from build123d import *

# Parameters (mm, degrees)
F0_W     = 70
F0_H     = 152.653071
F0_W_2   = 50.857146
F0_H_2   = 65.091088
F1_DEPTH = 8
F2_D     = 2
F2_DEPTH = 50
F3_R     = 10


with BuildPart() as f1:
    # F0 (on Top) → F1 (new body)
    with BuildSketch(Plane.XY):
        with Locations((0, 0.142402)):
            Rectangle(F0_W, F0_H)
        with Locations((0, -36.596865)):
            Rectangle(F0_W_2, F0_H_2, mode=Mode.SUBTRACT)
        with Locations((0, 36.596865)):
            Rectangle(F0_W_2, F0_H_2, mode=Mode.SUBTRACT)
    extrude(amount=F1_DEPTH)

    # F2
    with Locations(Plane(origin=(0, 0, 0), x_dir=(1, 0, 0), z_dir=(0, 0, -1))):
        with Locations((0, 2), (0, -2), (0, 73.713833), (0, -73.713833)):
            Hole(F2_D / 2, depth=F2_DEPTH)

    # F3
    f3_edges = [f1.edges().sort_by_distance(p)[0] for p in [
        (-35, 76.468938, 4),
        (35, 76.468938, 4),
        (-35, -76.184133, 4),
        (35, -76.184133, 4),
    ]]
    fillet(f3_edges, radius=F3_R)


solid = f1.part
Build history of the part. All positions in model axes, mm. A direction names the side the tool comes from. Round coordinates to 2 decimals unless told otherwise and drop trailing zeros. Write each loop counter-clockwise with the first axis right and the second up, starting at its lowest first coordinate (ties: lowest second). Pieces come first, ordered by that corner, then holes. Notation, with made-up numbers: M 58.5,-10.5 L 71.5,-10.5 A17 ccw 71.5,3.5 Z; hole C 34.25,-12.5 d5. An arc over 180 degrees is marked long. Answer as a JSON object with one key per item and string values. Group by question number.
(1) Which spindle directions (+Z, -Z, +X, -X, +Y, -Y) get a long thin tool onto all of the face, cutting with end or side? Do faces 4 (the flat face through (-25.429, -37, 4)), 5 (the flat face through (-35, -1, 4)). Say none if no direction does.
(2) Cut at A-A (y = 63). Give the cut face in (x, z).
(3) Flat gauge pin, fed straight in: pin 1 (12 mm diameter, centred on x = -15.5, y = 28.5, fed in from -Z). Where does the tip first touch, or does it go through?
(4) Cut at C-C (z = 2). Give the cut face in (x, y), and give its area (3 significant figures).
(5) Cut at D-D (x = 31.5). Give the cut face in (y, z), and give its area (3 significant figures).
(6) Drill centre lines: L1, parallel to Y at x = -7.5, z = 0.5; L2, parallel to X at y = 62, z = 7.5; L3, parallel to Y at x = 31, z = 4.25. Where is each one in solid material? Low to high.
(7) Mould opens along Y. For faces 1 (the flat face through (0, 4.051, 4)), 2 (the cylindrical face through (-32.15, 73.46, 4.06)), 3 (the flat face through (-3, 0, 0)) say: pulls with the +Y half, pulls with the -Y half, needs draft (parallel to the pull), parting line crosses it, or undercut.
(8) Cut at B-B (x = 14). Give the cut face in (y, z).
Responses:
{
 "1": {"face 4": "+Z, -Z", "face 5": "+Z, -Z, -X, +Y, -Y"},
 "2": {"outline": "M -35,0 L -25.43,0 L -25.43,8 L -35,8 Z; M 25.43,0 L 35,0 L 35,8 L 25.43,8 Z"},
 "3": {"pin 1": "passes through"},
 "4": {"outline": "M -35,-66.18 A10 ccw -25,-76.18 L 25,-76.18 A10 ccw 35,-66.18 L 35,66.47 A10 ccw 25,76.47 L -25,76.47 A10 ccw -35,66.47 Z; hole M -25.43,-69.14 L 25.43,-69.14 L 25.43,-4.05 L -25.43,-4.05 Z; hole M -25.43,4.05 L 25.43,4.05 L 25.43,69.14 L -25.43,69.14 Z; hole C 0,-73.71 d2; hole C 0,-2 d2; hole C 0,2 d2; hole C 0,73.71 d2", "area": "3,970 mm2"},
 "5": {"outline": "M -73.78,0 L 74.07,0 L 74.07,8 L -73.78,8 Z", "area": "1,180 mm2"},
 "6": {"L1": "y = -76.18 to -69.14, -4.05 to 4.05, 69.14 to 76.47", "L2": "x = -35 to -25.43, 25.43 to 35", "L3": "y = -74.18 to 74.47"},
 "7": {"face 1": "undercut", "face 2": "pulls with the +Y half", "face 3": "needs draft"},
 "8": {"outline": "M -76.18,0 L -69.14,0 L -69.14,8 L -76.18,8 Z; M -4.05,0 L 4.05,0 L 4.05,8 L -4.05,8 Z; M 69.14,0 L 76.47,0 L 76.47,8 L 69.14,8 Z"}
}
